Design review of the part built by this model. Coordinates are the model's own, in mm. Face numbers are marked on the shaded views. A direction names the side the tool comes from. Round coordinates to 2 decimals unless told otherwise and drop trailing zeros. Order: outer loops, then holes, each group sorted by start corner. A loop starts at its lowest first (then second) coordinate and runs counter-clockwise, first axis right, second up.
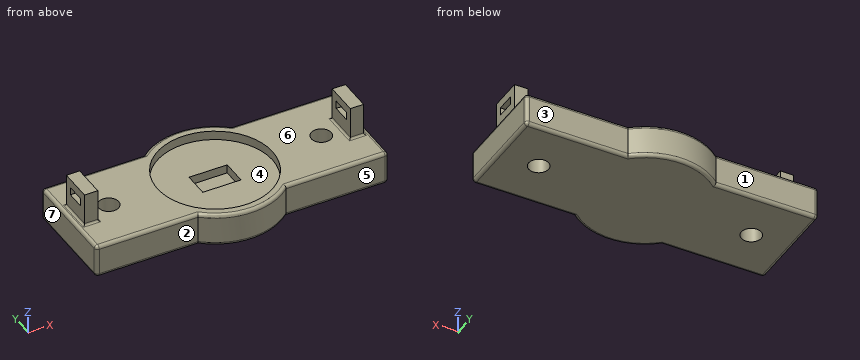
from build123d import *

# Parameters (mm, degrees)
PAD_DEPTH            = 5
SKETCH001_R          = 8.65
POCKET_DEPTH         = 1.38
SKETCH002_W          = 5.75
SKETCH002_H          = 3.8
POCKET001_DEPTH      = 1.32
SKETCH003_R          = 1.5
POCKET002_DEPTH      = 5.001
FILLET_R             = 0.5
SKETCH004_W          = 2
SKETCH004_H          = 5
PAD001_DEPTH         = 5
FILLET001_R          = 0.3
SKETCH005_W          = 2.8
SKETCH005_H          = 1.2
POCKET003_DEPTH      = 3.001
POCKET003_DEPTH_BACK = -41.001


with BuildPart() as part:
    # Sketch → Pad (new body)
    with BuildSketch(Plane.XY):
        with BuildLine():
            ThreePointArc((6.614378, 7.5), (0, 10), (-6.614378, 7.5))
            Line((-6.614378, 7.5), (-22, 7.5))
            Line((-22, 7.5), (-22, -7.5))
            Line((-22, -7.5), (-6.614378, -7.5))
            ThreePointArc((-6.614378, -7.5), (0, -10), (6.614378, -7.5))
            Line((22, -7.5), (6.614378, -7.5))
            Line((22, 7.5), (22, -7.5))
            Line((6.614378, 7.5), (22, 7.5))
        make_face()
    extrude(amount=PAD_DEPTH)

    # Sketch001 → Pocket (cut)
    with BuildSketch(Plane.XY.offset(5)):
        Circle(SKETCH001_R)
    extrude(amount=-POCKET_DEPTH, mode=Mode.SUBTRACT)

    # Sketch002 → Pocket001 (cut)
    with BuildSketch(Plane.XY.offset(3.62)):
        Rectangle(SKETCH002_W, SKETCH002_H)
    extrude(amount=-POCKET001_DEPTH, mode=Mode.SUBTRACT)

    # Sketch003 → Pocket002 (cut, through all)
    with BuildSketch(Plane.XY.offset(5)):
        with Locations((-16, 0)):
            Circle(SKETCH003_R)
        with Locations((16, 0)):
            Circle(SKETCH003_R)
    extrude(amount=-POCKET002_DEPTH, mode=Mode.SUBTRACT)

    # Fillet
    fillet_edges = [part.edges().sort_by_distance(p)[0] for p in [
        (-14.307189, 7.5, 0),
        (0, 10, 0),
        (14.307189, 7.5, 0),
        (22, 0, 0),
        (14.307189, -7.5, 0),
        (0, -10, 0),
        (-14.307189, -7.5, 0),
        (-22, 7.5, 2.5),
        (-22, 0, 0),
        (-22, -7.5, 2.5),
        (-22, 0, 5),
        (-14.307189, 7.5, 5),
        (0, 10, 5),
        (14.307189, 7.5, 5),
        (22, 7.5, 2.5),
        (22, 0, 5),
        (22, -7.5, 2.5),
        (14.307189, -7.5, 5),
        (0, -10, 5),
        (-14.307189, -7.5, 5),
    ]]
    fillet(fillet_edges, radius=FILLET_R)

    # Sketch004 → Pad001 (new body)
    with BuildSketch(Plane.XY.offset(5)):
        with Locations((-20, 0)):
            Rectangle(SKETCH004_W, SKETCH004_H)
        with Locations((20, 0)):
            Rectangle(SKETCH004_W, SKETCH004_H)
    extrude(amount=PAD001_DEPTH)

    # Fillet001
    fillet001_edges = [part.edges().sort_by_distance(p)[0] for p in [
        (-21, 0, 5),
        (-20, -2.5, 5),
        (20, -2.5, 5),
        (19, 0, 5),
        (-20, 2.5, 5),
        (-19, 0, 5),
        (20, 2.5, 5),
        (21, 0, 5),
    ]]
    fillet(fillet001_edges, radius=FILLET001_R)

    # Sketch005 → Pocket003 (cut, two sides)
    with BuildSketch(Plane.YZ.offset(-19)) as pocket003_sk:
        with Locations((0, 8.1)):
            Rectangle(SKETCH005_W, SKETCH005_H)
    extrude(amount=-POCKET003_DEPTH, mode=Mode.SUBTRACT)
    extrude(pocket003_sk.sketch, amount=-POCKET003_DEPTH_BACK, mode=Mode.SUBTRACT)


solid = part.part
1) To check wall thickness, follow line 1 along Y through (x, z) = (-16, 3.8); line 2 along X through (y, z) = (-1.75, 8); line 3 along Z through (x, y) = (6.5, 4.25). State the ranges of each line that lie inside material, in increasing order.
Results:
line 1: y = -7.5 to -1.5, 1.5 to 7.5
line 2: x = -21 to -19, 19 to 21
line 3: z = 0 to 3.62
2) For the marked faces 1, 2, 3 and 4, list the 3-axis set-ups (+Z, -Z, +X, -X, +Y, -Y) from which the entire face can be reached by the end or side of a thin tool; tool diameter is ignored.
Results:
face 1: +Z, -Z, -X, +Y
face 2: +Z, -Z, -X, -Y
face 3: +Z, -Z, +X, +Y
face 4: +Z
3) Take a section at A-A on z = 6.75. Give the boundary of the cut face in (x, y).
Results:
outline: (-21, -2.5) - (-19, -2.5) - (-19, 2.5) - (-21, 2.5) - close; (19, -2.5) - (21, -2.5) - (21, 2.5) - (19, 2.5) - close
4) Take a section at D-D on y = 6.5. Give the boundary of the cut face in (x, z), plus the area to 3 significant figures.
Results:
outline: (-22, 0.5) arc R0.5 ccw to (-21.5, 0) - (21.5, 0) arc R0.5 ccw to (22, 0.5) - (22, 4.5) arc R0.5 ccw to (21.5, 5) - (5.71, 5) - (5.71, 3.62) - (-5.71, 3.62) - (-5.71, 5) - (-21.5, 5) arc R0.5 ccw to (-22, 4.5) - close
area: 204 mm2
5) Take a section at B-B on x = 10. Give the boundary of the cut face in (y, z).
Results:
outline: (-7.5, 0.5) arc R0.5 ccw to (-7, 0) - (7, 0) arc R0.5 ccw to (7.5, 0.5) - (7.5, 4.5) arc R0.5 ccw to (7, 5) - (-7, 5) arc R0.5 ccw to (-7.5, 4.5) - close
6) Clearance check with flat-ended pins moving along their axes: P1, Ø2, axis at x = -14, z = 3.5, coming from the -Y side; P2, Ø4, axis at y = 4, z = 8.5, coming from the -X side; P3, Ø3, axis at x = 10.5, z = 1.5, coming from the +Y side. State where each tip first meets the part, or that it passes through.
Results:
P1: stops at y = -7.5
P2: stops at x = -21
P3: stops at y = 7.5
7) Take a section at C-C on x = -15. Give the boundary of the cut face in (y, z), plus the area to 3 significant figures.
Results:
outline: (-7.5, 0.5) arc R0.5 ccw to (-7, 0) - (-1.12, 0) - (-1.12, 5) - (-7, 5) arc R0.5 ccw to (-7.5, 4.5) - close; (1.12, 0) - (7, 0) arc R0.5 ccw to (7.5, 0.5) - (7.5, 4.5) arc R0.5 ccw to (7, 5) - (1.12, 5) - close
area: 63.6 mm2
8) The part is to be moulded in two halves that separate along X. For the marked faces 5, 6 and 7, say which applies: released by +X, released by -X, zero draft, split by the parting line, or undercut.
Results:
face 5: zero draft
face 6: undercut
face 7: released by -X
